The model under review builds one solid part; all positions refer to its coordinate system, in mm. A direction names the side the tool comes from. Coordinates: 2 decimals unless noted, no trailing zeros. Order: outer loops, then holes, each group sorted by start corner. A loop starts at its lowest first (then second) coordinate and runs counter-clockwise, first axis right, second up.
```python
from build123d import *

# Parameters (mm, degrees)
SKETCH1_R           = 10
BOSS_EXTRUDE1_DEPTH = 7
SKETCH2_R           = 10
BOSS_EXTRUDE2_DEPTH = 4
SKETCH3_R           = 7
BOSS_EXTRUDE3_DEPTH = 19
SKETCH4_R           = 3
CUT_EXTRUDE1_DEPTH  = 31
CHAMFER1_SIZE       = 0.5
CUT_EXTRUDE2_START  = 10.2
CUT_EXTRUDE2_DEPTH  = 5.8


with BuildPart() as part:
    # Sketch1 → Boss-Extrude1 (new body)
    with BuildSketch(Plane(origin=(0, 0, 0), x_dir=(0, 0, -1), z_dir=(1, 0, 0))):
        Circle(SKETCH1_R)
    extrude(amount=BOSS_EXTRUDE1_DEPTH)

    # Sketch2 → Boss-Extrude2 (add)
    with BuildSketch(Plane.ZY):
        with Locations((-0.336496213, 5)):
            Circle(SKETCH2_R)
    extrude(amount=BOSS_EXTRUDE2_DEPTH)

    # Sketch3 → Boss-Extrude3 (add)
    with BuildSketch(Plane.ZY.offset(4)):
        with Locations((-0.336496213, 5)):
            Circle(SKETCH3_R)
    extrude(amount=BOSS_EXTRUDE3_DEPTH)

    # Sketch4 → Cut-Extrude1 (cut, through all)
    with BuildSketch(Plane.ZY.offset(23)):
        with Locations((-0.336496213, 5)):
            Circle(SKETCH4_R)
    extrude(amount=-CUT_EXTRUDE1_DEPTH, mode=Mode.SUBTRACT)

    # Chamfer1
    chamfer1_edges = [part.edges().sort_by_distance(p)[0] for p in [
        (7, 5, -3.336496213),
        (-23, 5, -3.336496213),
    ]]
    chamfer(chamfer1_edges, length=CHAMFER1_SIZE)

    # Sketch5 → Cut-Extrude2 (cut, through all)
    with BuildSketch(Plane(origin=(0, 0, 0), x_dir=(1, 0, 0), z_dir=(0, 1, 0)).offset(CUT_EXTRUDE2_START)):
        with BuildLine():
            Line((-9, 2.836496213), (-26.986787276, 2.836496213))
            Line((-26.986787276, 2.836496213), (-26.986787276, -2.163503787))
            Line((-26.986787276, -2.163503787), (-9, -2.163503787))
            ThreePointArc((-9, -2.163503787), (-6.5, 0.336496213), (-9, 2.836496213))
        make_face()
    extrude(amount=CUT_EXTRUDE2_DEPTH, mode=Mode.SUBTRACT)


solid = part.part
```
(1) We need section C-C, the plane z = 8.75. Write out the cut boundary in (x, y).
A:
outline: (-4, 0.82) - (0, 0.82) - (0, -4.84) - (7, -4.84) - (7, 4.84) - (0, 4.84) - (0, 9.18) - (-4, 9.18) - close
(2) We need section B-B, the plane y = 5. Write out the cut boundary in (x, z), and give its area (3 significant figures).
A:
outline: (-23, -7.34) - (-4, -7.34) - (-4, -10.34) - (0, -10.34) - (0, -8.66) - (7, -8.66) - (7, -3.84) - (6.5, -3.34) - (-22.5, -3.34) - (-23, -3.84) - close; (-23, 3.16) - (-22.5, 2.66) - (6.5, 2.66) - (7, 3.16) - (7, 8.66) - (0, 8.66) - (0, 9.66) - (-4, 9.66) - (-4, 6.66) - (-23, 6.66) - close
area: 287 mm2
(3) Wall thickness on probe 1 along X at (y, z) = (13.5, 1.25); probe 2 along Y at (x, z) = (-16.5, -2.75); probe 3 along Y at (x, z) = (-3, 0.25): over which ranges is each line inside the solid? List them lowest first.
A:
probe 1: x = -4 to 0
probe 2: y = -1.57 to 3.22, 6.78 to 10.2
probe 3: y = -4.98 to 2.06, 7.94 to 14.98
(4) Machinability: for faces 1 (the face through (-13.37, -1.21, 2.89)), 2 (the face through (-15, 10.2, 0)), 3 (the face through (3.45, -9.76, 2.17)), 4 (the face through (0, -6, 0)), which of the approach directions +Z, -Z, +X, -X, +Y, -Y give a long, thin tool a straight path to every point of the face, cutting with its end or side? Answer none if there is none.
A:
face 1: -X
face 2: -X, +Y
face 3: +X
face 4: -X, -Y
(5) We need section A-A, the plane x = -15. Write out the cut boundary in (y, z), and give its area (3 significant figures).
A:
outline: (10.2, -2.84) - (10.2, 2.16) - (11.54, 2.16) arc R7 ccw (long way) to (11.54, -2.84) - close; hole circle Ø6 at (5, -0.34)
area: 117 mm2
(6) We need section D-D, the plane y = 0. Write out the cut boundary in (x, z).
A:
outline: (-23, -5.24) - (-4, -5.24) - (-4, -9) - (0, -9) - (0, -10) - (7, -10) - (7, 10) - (0, 10) - (0, 8.32) - (-4, 8.32) - (-4, 4.56) - (-23, 4.56) - close
(7) For pin 1 Ø2.5 at (x, z) = (-12, -0.5) entering from +Y; pin 2 Ø8 at (x, z) = (-13.5, 3.5) entering from -Y; pin 3 Ø1.1 at (x, y) = (-16.5, 10.5) entering from +Z; pin 4 Ø1.5 at (y, z) = (5.5, 1.5) entering from +X, all flat-tipped, find the tip position at first contact; note any pin that passes through.
A:
pin 1: stops at y = 10.2
pin 2: stops at y = -2
pin 3: stops at z = 4.61
pin 4: passes through
